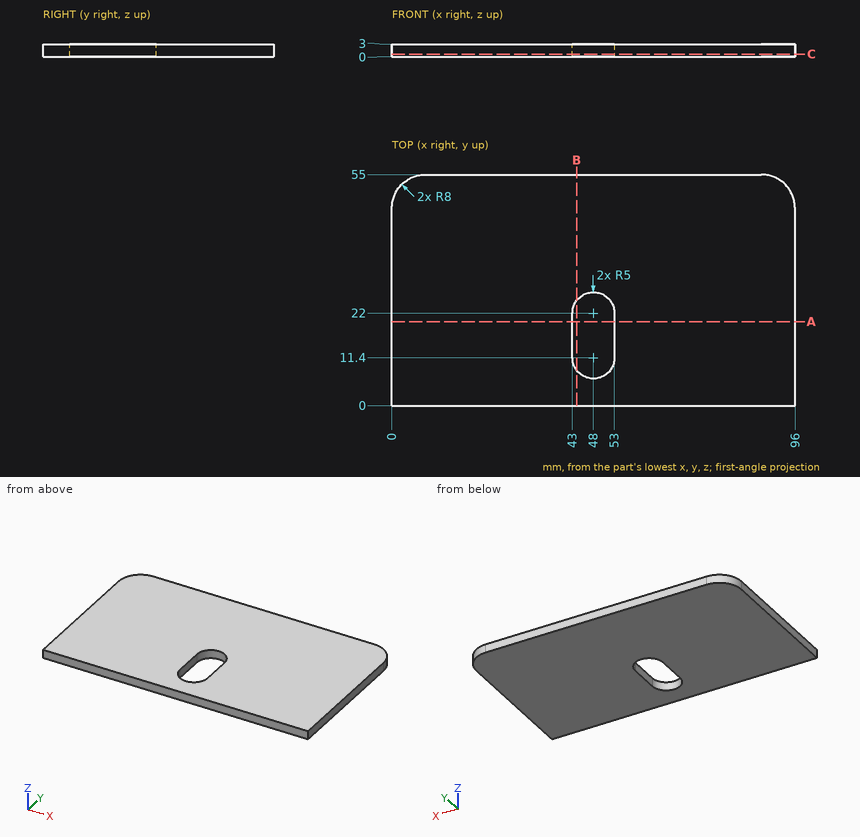
Geometry: see drawing. Coordinates: mm, zero at the bounding-box minimum. Coordinates: 2 decimals unless noted, no trailing zeros. Write each loop counter-clockwise with the first axis right and the second up, starting at its lowest first coordinate (ties: lowest second). Pieces come first, ordered by that corner, then holes.
1) Material intervals for line 1 along X through (y, z) = (14, 1.1); line 2 along X through (y, z) = (25, 1.1); line 3 along Y through (x, z) = (49, 1.1), sorted ascending.
2) Section C-C on z = 0.6. Output: boundary loops of the cut face in (x, y), and give its area (3 significant figures).
3) Section B-B on x = 44. Output: boundary loops of the cut face in (y, z), and give its area (3 significant figures).
4) Section A-A on y = 20. Output: boundary loops of the cut face in (x, z).
Check result:
1. line 1: x = 0 to 43, 53 to 96
1. line 2: x = 0 to 44, 52 to 96
1. line 3: y = 0 to 6.5, 26.9 to 55
2. outline: (0, 0) - (96, 0) - (96, 47) arc R8 ccw to (88, 55) - (8, 55) arc R8 ccw to (0, 47) - close; hole (43, 11.4) arc R5 ccw to (53, 11.4) - (53, 22) arc R5 ccw to (43, 22) - close
2. area: 5,070 mm2
3. outline: (0, 0) - (8.4, 0) - (8.4, 3) - (0, 3) - close; (25, 0) - (55, 0) - (55, 3) - (25, 3) - close
3. area: 115 mm2
4. outline: (0, 0) - (43, 0) - (43, 3) - (0, 3) - close; (53, 0) - (96, 0) - (96, 3) - (53, 3) - close
